The model under review builds one solid part; all positions refer to its coordinate system, in mm. A direction names the side the tool comes from. Coordinates: 2 decimals unless noted, no trailing zeros. Order: outer loops, then holes, each group sorted by start corner. A loop starts at its lowest first (then second) coordinate and runs counter-clockwise, first axis right, second up. Notation, with made-up numbers: M -38,74 L -8,74 A13 ccw -8,86 Z; hole C 45,17.5 d6. An arc over 180 degrees is marked long. Answer in a Markdown table with one row per item.
Autodesk Inventor part; units mm, degrees
ref_plane "YZ Plane" through (0, 0, 0) normal (1, 0, 0) x (0, 1, 0)
ref_plane "XZ Plane" through (0, 0, 0) normal (0, 1, 0) x (-1, 0, 0)
ref_plane "XY Plane" through (0, 0, 0) normal (0, 0, 1) x (1, 0, 0)
sketch "Sketch1" plane through (0, 0, 0) normal (0, 0, 1) x (1, 0, 0)
  line L0 (0, 0) -> (26.1364, 0)
  line L1 (26.1364, 0) -> (26.1364, 4.2728)
  line L2 (26.1364, 4.2728) -> (6.1364, 4.2728)
  line L3 (6.1364, 4.2728) -> (6.1364, 12.2728)
  line L4 (6.1364, 12.2728) -> (26.1364, 12.2728)
  line L5 (26.1364, 12.2728) -> (26.1364, 14.7274)
  line L6 (26.1364, 14.7274) -> (0, 14.7274)
  line L7 (0, 14.7274) -> (0, 0)
  line L8 (0, 14.7274) -> (0, 32.7274)
  arc A0 (19.9894, 33.187) -> (0, 32.7274) centre (10, 32.7274) ccw
  line L9 (19.9894, 33.187) -> (21, 14.7274)
  circle A1 centre (10, 32.7274) radius 2
  dimension "d0" = 20
  dimension "d1" = 8
  dimension "d3" = 4
  dimension "d4" = 10
  dimension "d5" = 18
  dimension "d7" = 19.9894
extrude "Extrusion1" add sketch "Sketch1" along normal blind 22
sketch "Sketch2" plane through (19.9894, 33.187, 22) normal (0.9985049, 0.0546629, 0) x (0, 0, -1)
  line L0 (1.8448, -6.1786) -> (1.8448, -17.437)
  line L1 (20.3448, -6.1786) -> (20.3448, -17.437)
  line L2 (20.3448, -17.437) -> (1.8448, -17.437)
  line L3 (1.8448, -6.1786) -> (1.8448, 10.563)
  line L4 (1.8448, 10.563) -> (20.3448, 10.563)
  line L5 (20.3448, 10.563) -> (20.3448, -6.1786)
  dimension "d14" = 28
  dimension "d17" = 18.5
extrude "Extrusion2" cut sketch "Sketch2" against normal through all
sketch "Sketch3" plane through (19.9894, 33.187, 22) normal (-0.9985049, -0.0546629, 0) x (0, 0, 1)
  line L0 (-20.3448, 0.1742) -> (-1.8448, 0.1742)
  line L1 (-1.8448, 0.1742) -> (-17.8448, 0.1742)
  line L2 (-17.8448, 0.1742) -> (-17.8448, -0.1891)
  line L3 (-17.8448, -0.1891) -> (-1.8448, -0.1891)
  line L4 (-1.8448, -0.1891) -> (-1.8448, 0.1742)
  point P0 (-22, -32.0447)
extrude "Extrusion3" cut sketch "Sketch3" against normal through all
sketch "Sketch4" plane through (21, 14.7274, 22) normal (0.9985049, 0.0546629, 0) x (0, 0, -1)
  point P0 (22, -13.5574)
sketch "Sketch5" plane through (0, 0, 22) normal (0, 0, 1) x (1, 0, 0)
  point P0 (0, 0)
sketch "Sketch6" plane through (0, 0, 0) normal (0, 0, -1) x (-1, 0, 0)
  point P0 (0, 0)
sketch "Sketch7" plane through (0, 0, 22) normal (0, 0, 1) x (1, 0, 0)
  point P0 (0, 0)
sketch "Sketch8" plane through (19.9894, 33.187, 22) normal (-0.9985049, -0.0546629, 0) x (0, 0, 1)
  point P0 (-22, -32.0447)
sketch "Sketch9" plane through (19.9894, 33.187, 22) normal (-0.9985049, -0.0546629, 0) x (0, 0, 1)
  line L0 (-20.3448, 0) -> (-20.3448, -17.437)
  line L1 (-20.3448, 0.1742) -> (-17.8448, 0.1742)
  line L2 (-20.3448, 0) -> (-17.8448, 0)
  line L3 (-17.8448, 0) -> (-17.8448, 0.1742)
  line L4 (-17.8448, 0.1742) -> (-20.3448, 0.1742)
  line L5 (-20.3448, 0.1742) -> (-20.3448, 0)
  point P0 (-22, -32.0447)
extrude "Extrusion4" cut sketch "Sketch9" against normal through all
properties part number "Maintients poullie v1"
(1) Take a section at C-C (y = 37). Write out the cut boundary in (x, z).
Report:
| item | result |
|---|---|
| outline | M 0.96,0 L 19.04,0 L 19.04,1.66 L 0.96,1.66 Z; M 0.96,20.16 L 19.04,20.16 L 19.04,22 L 0.96,22 Z |
(2) The part is to be moulded in two halves that separate along Z. For faces 1 (the flat face through (10.62, 15.21, 10.78)), 2 (the flat face through (10, 22, 22)), 3 (the cylindrical face through (10.923, 34.502, 0.816)), 4 (the flat face through (10, 22, 0)), say which applies: +Z half, -Z half, draft (parallel to the pull), parting line (faces both ways), or undercut.
Report:
| item | result |
|---|---|
| face 1 | undercut |
| face 2 | +Z half |
| face 3 | draft |
| face 4 | -Z half |
(3) Machinability: for faces 5 (the cylindrical face through (9.554, 42.717, 21.065)), 6 (the flat face through (24, 14.727, 11)), 7 (the flat face through (16, 4.273, 11)), which of the approach directions +Z, -Z, +X, -X, +Y, -Y give a long, thin tool a straight path to every point of the face, cutting with its end or side? Answer none if there is none.
Report:
| item | result |
|---|---|
| face 5 | +Z, -Z, +Y |
| face 6 | +Z, -Z, +X, +Y |
| face 7 | +Z, -Z, +X |
(4) Take a section at A-A (x = 23). Write out the cut boundary in (y, z), then the cut area to 3 significant figures.
Report:
| item | result |
|---|---|
| outline | M 0,0 L 4.27,0 L 4.27,22 L 0,22 Z; M 12.27,0 L 14.73,0 L 14.73,22 L 12.27,22 Z |
| area | 148 mm^2 |
(5) To check wall thickness, follow line 1 (Y direction, x = 10, z = 1.1); line 2 (Z direction, x = 20.25, y = 25); line 3 (Y direction, x = 24.5, z = 17.5). State the ranges of each line that lie inside material, in increasing order. Write a range as [from, to].
Report:
| item | result |
|---|---|
| line 1 | [0, 4.27], [12.27, 30.73], [34.73, 42.73] |
| line 2 | [0, 1.66], [20.16, 22] |
| line 3 | [0, 4.27], [12.27, 14.73] |
(6) Take a section at B-B (z = 3.25). Write out the cut boundary in (x, y).
Report:
| item | result |
|---|---|
| outline | M 0,0 L 26.14,0 L 26.14,4.27 L 6.14,4.27 L 6.14,12.27 L 26.14,12.27 L 26.14,14.73 L 21,14.73 L 20.94,15.78 L 0,14.63 Z |
(7) Insertion check: P1, Ø8, axis at x = 23.5, z = 7, coming from the +Y side. The pin has a flat end and moves straight along its axis. Give the tip position at first contact, or say it passes through.
Report:
| item | result |
|---|---|
| P1 | y = 15.78 |
(8) Take a section at D-D (x = 10). Write out the cut boundary in (y, z).
Report:
| item | result |
|---|---|
| outline | M 0,0 L 4.27,0 L 4.27,22 L 0,22 Z; M 12.27,0 L 30.73,0 L 30.73,1.66 L 15.18,1.66 L 15.18,20.16 L 30.73,20.16 L 30.73,22 L 12.27,22 Z; M 34.73,0 L 42.73,0 L 42.73,1.66 L 34.73,1.66 Z; M 34.73,20.16 L 42.73,20.16 L 42.73,22 L 34.73,22 Z |
